```python
from build123d import *

# Parameters (mm, degrees)
F1_DEPTH = 25.4
F2_R     = 5.08
F3_D     = 5.1054


with BuildPart() as f1:
    # F0 (on Right) → F1 (new body)
    with BuildSketch(Plane.YZ):
        Polygon((50.8, -21.0420489686), (50.8, 21.0420489686), (21.0420489686, 50.8), (-21.0420489686, 50.8), (-50.8, 21.0420489686), (-50.8, -21.0420489686), (-21.0420489686, -50.8), (21.0420489686, -50.8), align=None)
    extrude(amount=F1_DEPTH)

    # F2
    f2_edges = [f1.edges().sort_by_distance(p)[0] for p in [
        (25.4, -35.921024, 35.921024),
        (25.4, -50.8, 0),
        (25.4, -35.921024, -35.921024),
        (25.4, 0, -50.8),
        (25.4, 35.921024, -35.921024),
        (25.4, 50.8, 0),
        (25.4, 35.921024, 35.921024),
        (25.4, 0, 50.8),
    ]]
    fillet(f2_edges, radius=F2_R)

    # F3 (through all)
    with Locations(Plane(origin=(0, 0, 0), x_dir=(0, 1, 0), z_dir=(-1, 0, 0))):
        with Locations((0, 0)):
            Hole(F3_D / 2)


solid = f1.part
```
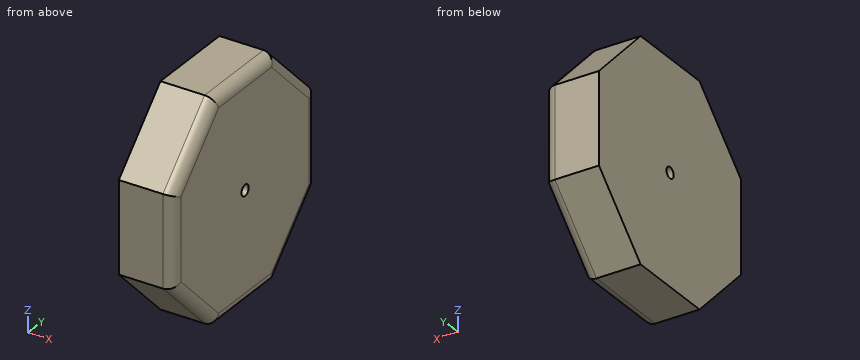
CAD build for the part. Positions are in the model's coordinates, mm. Round coordinates to 2 decimals unless told otherwise and drop trailing zeros. Write each loop counter-clockwise with the first axis right and the second up, starting at its lowest first coordinate (ties: lowest second). Pieces come first, ordered by that corner, then holes. Notation, with made-up numbers: (24, 19.5) - (79, 19.5) arc R19 ccw to (79, 46.5) - close; hole circle Ø11 at (-35.5, -20). An arc over 180 degrees is marked (long way). Return JSON: item names as keys, results as strings. Group by question number.
Item 1: Band-saw the part on C-C on x = 11.5. List the corners of the cut face in (y, z), plus the area to 3 significant figures.
Item 2: Band-saw the part on D-D on x = 21.75. List the corners of the cut face in (y, z).
Item 3: Probe probe 1 along Z at (x, y) = (18.75, 0); probe 2 along Y at (x, z) = (20.75, -20); probe 3 along Z at (x, y) = (1.5, -1). List the from-to ranges inside material, lowest first.
Item 4: Flat gauge pins, fed straight in: pin 1 Ø4.5 at (y, z) = (0, 0) entering from -X; pin 2 Ø2 at (x, z) = (9.5, 26.5) entering from -Y; pin 3 Ø2 at (y, z) = (-4, 35.5) entering from -X. Where does each tip first touch, or does it go through?
Item 5: Band-saw the part on A-A on z = 0. List the corners of the cut face in (x, y).
Resolved:
{
 "1": {"outline": "(-50.8, -21.04) - (-21.04, -50.8) - (21.04, -50.8) - (50.8, -21.04) - (50.8, 21.04) - (21.04, 50.8) - (-21.04, 50.8) - (-50.8, 21.04) - close; hole circle Ø5.11 at (0, 0)", "area": "8,530 mm²"},
 "2": {"outline": "(-50.59, -20.96) - (-20.96, -50.59) - (20.96, -50.59) - (50.59, -20.96) - (50.59, 20.96) - (20.96, 50.59) - (-20.96, 50.59) - (-50.59, 20.96) - close; hole circle Ø5.11 at (0, 0)"},
 "3": {"probe 1": "z = -50.8 to -2.55, 2.55 to 50.8", "probe 2": "y = -50.78 to 50.78", "probe 3": "z = -50.8 to -2.35, 2.35 to 50.8"},
 "4": {"pin 1": "passes through", "pin 2": "stops at y = -46.34", "pin 3": "stops at x = 0"},
 "5": {"outline": "(0, -50.8) - (20.32, -50.8) arc R5.08 ccw to (25.4, -45.72) - (25.4, -2.55) - (0, -2.55) - close; (0, 2.55) - (25.4, 2.55) - (25.4, 45.72) arc R5.08 ccw to (20.32, 50.8) - (0, 50.8) - close"}
}
